For this review, take the finished solid that the model builds, in its own axes (mm). Face numbers are marked on the shaded views. A direction names the side the tool comes from. Round coordinates to 2 decimals unless told otherwise and drop trailing zeros. Order: outer loops, then holes, each group sorted by start corner. A loop starts at its lowest first (then second) coordinate and runs counter-clockwise, first axis right, second up. Notation, with made-up numbers: (48, 37.5) -> (55, 37.5) arc R22 cw to (55, 61.5) -> close; hole circle Ø1 at (4, 2.25). An arc over 180 degrees is marked (long way). Use a Markdown table: item, result. Add a question column.
1) Machinability: for the marked faces 1, 2, 3 and 4, which of the approach directions +Z, -Z, +X, -X, +Y, -Y give a long, thin tool a straight path to every point of the face, cutting with its end or side? Answer none if there is none.
2) Clearance check with flat-ended pins moving along their axes: P1, Ø1, axis at x = -2, z = 34.5, coming from the +Y side; P2, Ø7, axis at x = 0, z = 38, coming from the -Y side; P3, Ø8, axis at y = -4, z = 4, coming from the +X side; P4, Ø5, axis at x = 5, y = -0.5, coming from the -Z side. State where each tip first meets the part, or that it passes through.
3) Wall thickness on line 1 along Z through (x, y) = (4, -4); line 2 along Y through (x, z) = (0.25, 16); line 3 along X through (y, z) = (3, 2.5): over which ranges is each line inside the solid? List them lowest first. Write a range as [from, to].
4) Consider section A-A (x = 0). State the section outline as (y, z) points.
5) Consider section D-D (z = 23.5). State the section outline as (x, y) points, plus the area to 3 significant figures.
6) Consider section C-C (z = 38). State the section outline as (x, y) points.
7) Consider section B-B (y = 0). State the section outline as (x, z) points, plus the area to 3 significant figures.
```python
from build123d import *

# Parameters (mm, degrees)
F0_R     = 4
F1_DEPTH = 41
F2_DEPTH = 3
F0_R_2   = 7
F3_DEPTH = 3
F5_DEPTH = 10
F6_SIZE2 = 0.5
F6_SIZE  = 0.5
F7_SIZE2 = 0.5
F7_SIZE  = 0.5
F8_SIZE2 = 0.5
F8_SIZE  = 0.5


with BuildPart() as f1:
    # F0 (on Top) → F1 (new body)
    with BuildSketch(Plane.XY):
        Circle(F0_R)
    extrude(amount=F1_DEPTH)

    # F0 (on Top) → F2 (join)
    with BuildSketch(Plane.XY):
        Circle(F0_R)
    extrude(amount=-F2_DEPTH)

    # F0 (on Top) → F3 (join)
    with BuildSketch(Plane.XY):
        Circle(F0_R_2)
        Circle(F0_R, mode=Mode.SUBTRACT)
    extrude(amount=F3_DEPTH)

    # F4 (on face) → F5 (cut)
    with BuildSketch(Plane.XY.offset(41)):
        Polygon((4.573411, -5.26242), (4.573411, -2.5), (0, -2.5), (-4.510589, -2.5), (-4.510589, -5.26242), align=None)
    extrude(amount=-F5_DEPTH, mode=Mode.SUBTRACT)

    # F6
    f6_edges = [f1.edges().sort_by_distance(p)[0] for p in [
        (-7, 0, 3),
    ]]
    chamfer(f6_edges, length=F6_SIZE, length2=F6_SIZE2)

    # F7
    f7_edges = [f1.edges().sort_by_distance(p)[0] for p in [
        (-7, 0, 0),
    ]]
    chamfer(f7_edges, length=F7_SIZE, length2=F7_SIZE2)

    # F8
    f8_edges = [f1.edges().sort_by_distance(p)[0] for p in [
        (-4, 0, -3),
    ]]
    chamfer(f8_edges, length=F8_SIZE, length2=F8_SIZE2)


solid = f1.part
```
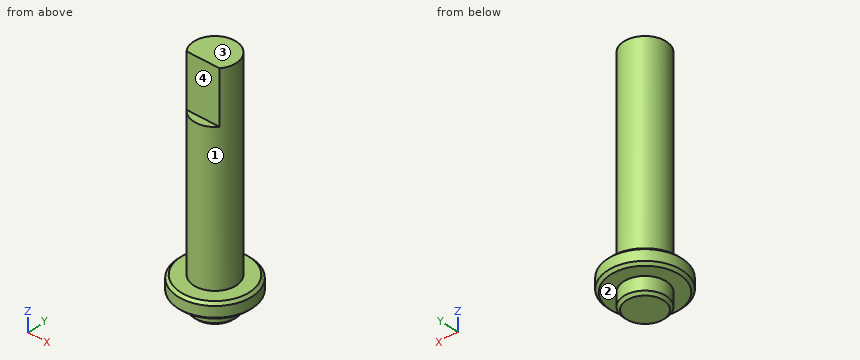
Results list:
| question | item | result |
|---|---|---|
| 1 | face 1 | +Z |
| 1 | face 2 | -Z |
| 1 | face 3 | +Z, +X, -X, +Y, -Y |
| 1 | face 4 | +Z, +X, -X, -Y |
| 2 | P1 | y = 3.71 |
| 2 | P2 | y = -2.5 |
| 2 | P3 | x = 6.99 |
| 2 | P4 | z = -3 |
| 3 | line 1 | [0, 3] |
| 3 | line 2 | [-3.99, 3.99] |
| 3 | line 3 | [-6.32, 6.32] |
| 4 | outline | (-7, 0.5) -> (-6.5, 0) -> (-4, 0) -> (-4, -2.5) -> (-3.5, -3) -> (3.5, -3) -> (4, -2.5) -> (4, 0) -> (6.5, 0) -> (7, 0.5) -> (7, 2.5) -> (6.5, 3) -> (4, 3) -> (4, 41) -> (-2.5, 41) -> (-2.5, 31) -> (-4, 31) -> (-4, 3) -> (-6.5, 3) -> (-7, 2.5) -> close |
| 5 | outline | circle Ø8 at (0, 0) |
| 5 | area | 50.3 mm2 |
| 6 | outline | (-3.12, -2.5) -> (3.12, -2.5) arc R4 ccw (long way) to start |
| 7 | outline | (-7, 0.5) -> (-6.5, 0) -> (-4, 0) -> (-4, -2.5) -> (-3.5, -3) -> (3.5, -3) -> (4, -2.5) -> (4, 0) -> (6.5, 0) -> (7, 0.5) -> (7, 2.5) -> (6.5, 3) -> (4, 3) -> (4, 41) -> (-4, 41) -> (-4, 3) -> (-6.5, 3) -> (-7, 2.5) -> close |
| 7 | area | 369 mm2 |
